Work out the finished part from the listing and answer in its coordinate system (mm). Face numbers are marked on the shaded views. A direction names the side the tool comes from. Round coordinates to 2 decimals unless told otherwise and drop trailing zeros. Write each loop counter-clockwise with the first axis right and the second up, starting at its lowest first coordinate (ties: lowest second). Pieces come first, ordered by that corner, then holes. Notation, with made-up numbers: M 64,6.5 L 123,6.5 A29 ccw 123,35.5 Z; hole C 17.5,84.25 d6. An arc over 180 degrees is marked long. Answer in a Markdown table with one row per item.
```python
from build123d import *

# Parameters (mm, degrees)
SKETCH1_W           = 160
SKETCH1_H           = 61
BOSS_EXTRUDE1_DEPTH = 2
SKETCH2_W           = 160
SKETCH2_H           = 2
BOSS_EXTRUDE2_DEPTH = 17
SKETCH3_W           = 156
SKETCH3_H           = 2
BOSS_EXTRUDE3_DEPTH = 17
SKETCH4_W           = 70
SKETCH4_H           = 2
BOSS_EXTRUDE4_DEPTH = 42
SKETCH5_W           = 4
SKETCH5_H           = 8
CUT_EXTRUDE1_DEPTH  = 39
FILLET1_R           = 2
SKETCH6_W           = 2
SKETCH6_H           = 42
BOSS_EXTRUDE5_DEPTH = 17
SKETCH9_W           = 66
SKETCH9_H           = 2
BOSS_EXTRUDE6_DEPTH = 17


with BuildPart() as part:
    # Sketch1 → Boss-Extrude1 (new body)
    with BuildSketch(Plane(origin=(0, 0, 0), x_dir=(1, 0, 0), z_dir=(0, 1, 0))):
        with Locations((80, -30.5)):
            Rectangle(SKETCH1_W, SKETCH1_H)
    extrude(amount=BOSS_EXTRUDE1_DEPTH)

    # Sketch2 → Boss-Extrude2 (add)
    with BuildSketch(Plane(origin=(0, 2, 0), x_dir=(1, 0, 0), z_dir=(0, 1, 0))):
        with Locations((80, -1)):
            Rectangle(SKETCH2_W, SKETCH2_H)
    extrude(amount=BOSS_EXTRUDE2_DEPTH)

    # Sketch3 → Boss-Extrude3 (add)
    with BuildSketch(Plane(origin=(0, 2, 0), x_dir=(1, 0, 0), z_dir=(0, 1, 0))):
        Polygon((0, -2), (0, -61), (2, -61), (2, -59), (2, -2), align=None)
        Polygon((158, -59), (158, -61), (160, -61), (160, -2), (158, -2), align=None)
        with Locations((80, -60)):
            Rectangle(SKETCH3_W, SKETCH3_H)
    extrude(amount=BOSS_EXTRUDE3_DEPTH)

    # Sketch4 → Boss-Extrude4 (add)
    with BuildSketch(Plane(origin=(0, 0, 0), x_dir=(-1, 0, 0), z_dir=(0, 0, -1))):
        with Locations((-80, 1)):
            Rectangle(SKETCH4_W, SKETCH4_H)
    extrude(amount=BOSS_EXTRUDE4_DEPTH)

    # Sketch5 → Cut-Extrude1 (cut)
    with BuildSketch(Plane(origin=(0, 0, 0), x_dir=(-1, 0, 0), z_dir=(0, 0, -1))):
        with Locations((-55.116937283, 19)):
            Rectangle(SKETCH5_W, SKETCH5_H)
    extrude(amount=-CUT_EXTRUDE1_DEPTH, mode=Mode.SUBTRACT)

    # Fillet1
    fillet1_edges = [part.edges().sort_by_distance(p)[0] for p in [
        (53.116937283, 19, 1),
        (57.116937283, 19, 1),
    ]]
    fillet(fillet1_edges, radius=FILLET1_R)

    # Sketch6 → Boss-Extrude5 (add)
    with BuildSketch(Plane(origin=(0, 2, 0), x_dir=(1, 0, 0), z_dir=(0, 1, 0))):
        with Locations((114, 21)):
            Rectangle(SKETCH6_W, SKETCH6_H)
    extrude(amount=BOSS_EXTRUDE5_DEPTH)

    # Sketch9 → Boss-Extrude6 (add)
    with BuildSketch(Plane(origin=(0, 2, 0), x_dir=(1, 0, 0), z_dir=(0, 1, 0))):
        Polygon((47, 42), (45, 42), (45, 0), (47, 0), (47, 40), align=None)
        with Locations((80, 41)):
            Rectangle(SKETCH9_W, SKETCH9_H)
    extrude(amount=BOSS_EXTRUDE6_DEPTH)


solid = part.part
```
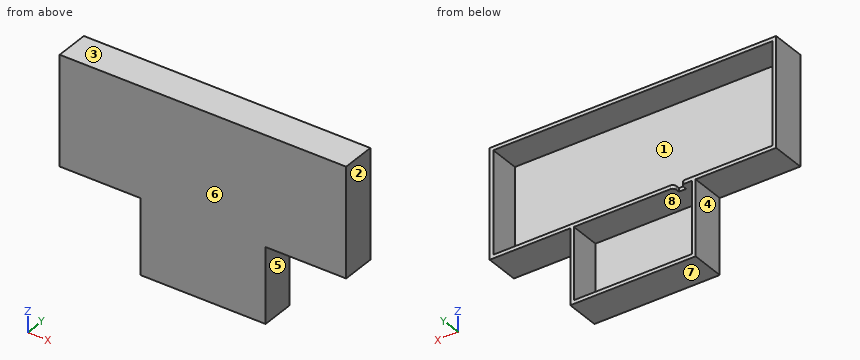
1. Determine the mould class of the marked faces 1, 2 and 3 for opening direction X: released by +X, released by -X, zero draft, split by the parting line, or undercut.
Calculated:
| item | result |
|---|---|
| face 1 | undercut |
| face 2 | released by +X |
| face 3 | zero draft |
2. The part is cut by section D-D (x = 148). Determine the outline of the cut face in (y, z), plus the area to 3 significant figures.
Calculated:
| item | result |
|---|---|
| outline | M 0,0 L 19,0 L 19,2 L 2,2 L 2,59 L 19,59 L 19,61 L 0,61 Z |
| area | 190 mm² |
3. Consider line 1 along Z through (x, y) = (78, 10.75); line 2 along X through (y, z) = (7.5, -33); line 3 along Z through (x, y) = (35, 15). Determine where each line is inside the solid, lowest interval first. Write a range as from..to.
Calculated:
| item | result |
|---|---|
| line 1 | z = -42..-40, 0..2, 59..61 |
| line 2 | x = 45..47, 113..115 |
| line 3 | z = 0..2, 59..61 |
4. The part is cut by section B-B (x = 63). Determine the outline of the cut face in (y, z), plus the area to 3 significant figures.
Calculated:
| item | result |
|---|---|
| outline | M 0,-42 L 19,-42 L 19,-40 L 2,-40 L 2,0 L 19,0 L 19,2 L 2,2 L 2,59 L 19,59 L 19,61 L 0,61 Z |
| area | 308 mm² |
5. A tool of negligible diameter and unlimited length cuts with its end or side. For the marked faces 4, 5, 6, 7 and 8, from which of +Z, -Z, +X, -X, +Y, -Y can it reach the whole face along a straight path? Write none if from no direction.
Calculated:
| item | result |
|---|---|
| face 4 | -Z, -X, +Y, -Y |
| face 5 | -Z, +X, +Y, -Y |
| face 6 | +Z, -Z, +X, -X, -Y |
| face 7 | -Z, +X, -X, +Y, -Y |
| face 8 | +Y |
6. Given pin 1 (5 mm diameter, centred on y = 7.5, z = -27.5, fed in from +X); pin 2 (5.5 mm diameter, centred on x = 128, y = 14, fed in from -Z); pin 3 (5.5 mm diameter, centred on y = 13.5, z = -22, fed in from -X), each flat-ended and moving along its own axis, determine where each tip first touches the part or whether it passes through.
Calculated:
| item | result |
|---|---|
| pin 1 | stops at x = 115 |
| pin 2 | stops at z = 0 |
| pin 3 | stops at x = 45 |
7. The part is cut by section A-A (y = 4.25). Determine the outline of the cut face in (x, z), plus the area to 3 significant figures.
Calculated:
| item | result |
|---|---|
| outline | M 0,0 L 45,0 L 45,-42 L 115,-42 L 115,0 L 160,0 L 160,61 L 0,61 Z; hole M 2,2 L 158,2 L 158,59 L 2,59 Z; hole M 47,-40 L 113,-40 L 113,0 L 47,0 Z |
| area | 1,170 mm² |
8. The part is cut by section C-C (z = -27.5). Determine the outline of the cut face in (x, y), plus the area to 3 significant figures.
Calculated:
| item | result |
|---|---|
| outline | M 45,0 L 115,0 L 115,19 L 113,19 L 113,2 L 47,2 L 47,19 L 45,19 Z |
| area | 208 mm² |
